```python
from build123d import *

# Parameters (mm, degrees)
BOSS_EXTRUDE1_DEPTH                        = 20
SKETCH2_R                                  = 1.5
CUT_EXTRUDE1_DEPTH                         = 6
MIRROR1_AT_THE_SECOND_PLANE_COPY_1_SKETC_R = 1.5
MIRROR1_AT_THE_SECOND_PLANE_COPY_1_DEPTH   = 6


with BuildPart() as part:
    # Sketch1 → Boss-Extrude1 (new, symmetric)
    with BuildSketch(Plane(origin=(0, 0, 0), x_dir=(1, 0, 0), z_dir=(0, 1, 0))):
        Polygon((2.886751346, 0), (1.443375673, 2.5), (-1.443375673, 2.5), (-2.886751346, 0), (-1.443375673, -2.5), (1.443375673, -2.5), align=None)
    extrude(amount=BOSS_EXTRUDE1_DEPTH, both=True)

    # Sketch2 → Cut-Extrude1 (cut)
    with BuildSketch(Plane(origin=(0, 20, 0), x_dir=(1, 0, 0), z_dir=(0, 1, 0))):
        with Locations(Location((0, 0, 0), (0, 0, 270))):
            Circle(SKETCH2_R)
    cut_extrude1 = extrude(amount=-CUT_EXTRUDE1_DEPTH, mode=Mode.SUBTRACT)

    # Mirror1: Cut-Extrude1 across plane
    add(cut_extrude1.mirror(Plane(origin=(0, 0, 0), x_dir=(0, 0, 1), z_dir=(1, 0, 0))), mode=Mode.SUBTRACT)

    # Mirror1 at the second plane: Cut-Extrude1 across plane
    add(cut_extrude1.mirror(Plane.ZX), mode=Mode.SUBTRACT)

    # Mirror1 at the second plane copy 1 sketc → Mirror1 at the second plane copy 1 (cut)
    with BuildSketch(Plane(origin=(0, -20, 0), x_dir=(-1, 0, 0), z_dir=(0, -1, 0))):
        with Locations(Location((0, 0, 0), (0, 0, 270))):
            Circle(MIRROR1_AT_THE_SECOND_PLANE_COPY_1_SKETC_R)
    extrude(amount=-MIRROR1_AT_THE_SECOND_PLANE_COPY_1_DEPTH, mode=Mode.SUBTRACT)


solid = part.part
```
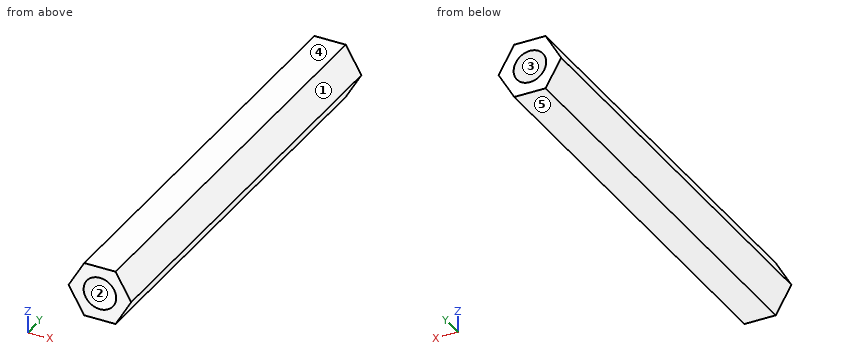
Read the model definition and answer for the solid it produces. Units are mm, in the model's axes. Face numbers are marked on the shaded views. A direction names the side the tool comes from. Coordinates: 2 decimals unless noted, no trailing zeros. Write each loop counter-clockwise with the first axis right and the second up, starting at its lowest first coordinate (ties: lowest second). Pieces come first, ordered by that corner, then holes. Notation, with made-up numbers: (-24.5, 6.25) - (11.5, 6.25) arc R35 ccw to (11.5, 45.25) - close; hole circle Ø11 at (17.25, 22). An arc over 180 degrees is marked (long way). Answer as a JSON object with one key per item and string values. Group by question number.
1. A cutting plane is placed at C-C (z = 0.75). Determine the outline of the cut face in (x, y), plus the area to 3 significant figures.
2. The mould has two halves that part along Z. Classify the marked faces 3, 4 and 5: +Z half, -Z half, draft (parallel to the pull), parting line (faces both ways), or undercut.
3. Consider L1, parallel to Y at x = 0.5, z = 1; L2, parallel to X at y = 7.5, z = -1.4; L3, parallel to X at y = -10, z = -2. Determine where each line is inside the solid, lowest interval first. Write a range as [from, to].
4. A cutting plane is placed at D-D (y = 7). Determine the outline of the cut face in (x, z), plus the area to 3 significant figures.
5. Each of these flat-tipped pins is pushed along its axis until it touches: P1, Ø1.8, axis at x = 0, z = 0, coming from the +Y side; P2, Ø1.5, axis at y = 14, z = -1.5, coming from the -X side. Where does it stop, or does it pass through?
6. Which of the six approach directions +Z, -Z, +X, -X, +Y, -Y give full straight-line access (tool end or side, diameter ignored) to the marked faces 1 and 2?
7. A cutting plane is placed at A-A (y = -14.5). Determine the outline of the cut face in (x, z).
8. A cutting plane is placed at B-B (x = 0). Determine the outline of the cut face in (y, z), plus the area to 3 significant figures.
Worked out:
{
 "1": {"outline": "(-2.45, -20) - (-1.3, -20) - (-1.3, -14) - (1.3, -14) - (1.3, -20) - (2.45, -20) - (2.45, 20) - (1.3, 20) - (1.3, 14) - (-1.3, 14) - (-1.3, 20) - (-2.45, 20) - close", "area": "165 mm²"},
 "2": {"face 3": "undercut", "face 4": "+Z half", "face 5": "-Z half"},
 "3": {"L1": "y = [-14, 14]", "L2": "x = [-2.08, 2.08]", "L3": "x = [-1.73, 1.73]"},
 "4": {"outline": "(-2.89, 0) - (-1.44, -2.5) - (1.44, -2.5) - (2.89, 0) - (1.44, 2.5) - (-1.44, 2.5) - close", "area": "21.7 mm²"},
 "5": {"P1": "stops at y = 14", "P2": "stops at x = -2.45"},
 "6": {"face 1": "+Z, +X, +Y, -Y", "face 2": "-Y"},
 "7": {"outline": "(-2.89, 0) - (-1.44, -2.5) - (1.44, -2.5) - (2.89, 0) - (1.44, 2.5) - (-1.44, 2.5) - close; hole circle Ø3 at (0, 0)"},
 "8": {"outline": "(-20, -2.5) - (20, -2.5) - (20, -1.5) - (14, -1.5) - (14, 1.5) - (20, 1.5) - (20, 2.5) - (-20, 2.5) - (-20, 1.5) - (-14, 1.5) - (-14, -1.5) - (-20, -1.5) - close", "area": "164 mm²"}
}
